Source: CAD feature listing. Evaluate the final solid. Frame: model axes, mm. A direction names the side the tool comes from. Give positions to 0.01 mm unless a question says otherwise; leave off trailing zeros. Order: outer loops, then holes, each group sorted by start corner. A loop starts at its lowest first (then second) coordinate and runs counter-clockwise, first axis right, second up.
from build123d import *

# Parameters (mm, degrees)
F2_R     = 20
F3_DEPTH = 20
F5_DEPTH = 15


with BuildPart() as f1:
    # F0 (on Front) → F1 (revolve)
    with BuildSketch(Plane.XZ):
        Polygon((29.861114, 20), (9.861114, 20), (9.861114, 65.476191), (29.861114, 65.476191), (29.861114, 90.476191), (0, 90.476191), (0, 0), (29.861114, 0), align=None)
    revolve(axis=Axis((0, 0, 45.238095), (0, 0, -1)))

    # F2 (on face) → F3 (cut)
    with BuildSketch(Plane.XY.offset(90.476191)):
        Circle(F2_R)
    extrude(amount=-F3_DEPTH, mode=Mode.SUBTRACT)

    # F4 (on face) → F5 (cut)
    with BuildSketch(Plane.XY.offset(90.476191)):
        with BuildLine():
            ThreePointArc((-3.013717, 17.091636), (0, 17.355302), (3.013717, 17.091636))
            Line((3.013717, 17.091636), (6.241417, 35.396835))
            ThreePointArc((6.241417, 35.396835), (0, 35.942888), (-6.241417, 35.396835))
            Line((-6.241417, 35.396835), (-3.013717, 17.091636))
        make_face()
        with BuildLine():
            Line((-33.775267, 12.293192), (-16.308649, 5.935863))
            ThreePointArc((-16.308649, 5.935863), (-15.030132, 8.677651), (-13.294933, 11.155773))
            Line((-13.294933, 11.155773), (-27.53385, 23.103643))
            ThreePointArc((-27.53385, 23.103643), (-31.127454, 17.971444), (-33.775267, 12.293192))
        make_face()
        with BuildLine():
            Line((-27.53385, -23.103643), (-13.294933, -11.155773))
            ThreePointArc((-13.294933, -11.155773), (-15.030132, -8.677651), (-16.308649, -5.935863))
            Line((-16.308649, -5.935863), (-33.775267, -12.293192))
            ThreePointArc((-33.775267, -12.293192), (-31.127454, -17.971444), (-27.53385, -23.103643))
        make_face()
        with BuildLine():
            Line((6.241417, -35.396835), (3.013717, -17.091636))
            ThreePointArc((3.013717, -17.091636), (0, -17.355302), (-3.013717, -17.091636))
            Line((-3.013717, -17.091636), (-6.241417, -35.396835))
            ThreePointArc((-6.241417, -35.396835), (0, -35.942888), (6.241417, -35.396835))
        make_face()
        with BuildLine():
            Line((33.775267, -12.293192), (16.308649, -5.935863))
            ThreePointArc((16.308649, -5.935863), (15.030132, -8.677651), (13.294933, -11.155773))
            Line((13.294933, -11.155773), (27.53385, -23.103643))
            ThreePointArc((27.53385, -23.103643), (31.127454, -17.971444), (33.775267, -12.293192))
        make_face()
        with BuildLine():
            Line((27.53385, 23.103643), (13.294933, 11.155773))
            ThreePointArc((13.294933, 11.155773), (15.030132, 8.677651), (16.308649, 5.935863))
            Line((16.308649, 5.935863), (33.775267, 12.293192))
            ThreePointArc((33.775267, 12.293192), (31.127454, 17.971444), (27.53385, 23.103643))
        make_face()
    extrude(amount=-F5_DEPTH, mode=Mode.SUBTRACT)


solid = f1.part
(1) Draft query along Z for faces 4 (the flat face through (-24, 0, 90.476)), 5 (the flat face through (7.1, -7.1, 65.476)), 6 (the flat face through (4.317, 24.484, 83.081)). Return one class per face: +Z half, -Z half, draft (parallel to the pull), parting line (faces both ways), or undercut.
(2) Section A-A, the plane x = 12.5. Return loops of the section in (y, z), plus the area to 3 significant figures.
(3) Pin query (flat end, axial travel): pin 1 Ø10 at (y, z) = (10, 46.5) entering from -X; pin 2 Ø3.5 at (x, y) = (23.5, -12) entering from +Z; pin 3 Ø6 at (x, z) = (-11, 52) entering from -Y. Return the tip coordinate at first contact, or that it passes through.
(4) Section C-C, the plane y = 0. Return loops of the section in (x, z).
(5) Section B-B, the plane y = 14. Return loops of the section in (x, z), plus the area to 3 significant figures.
(6) Access query for faces 1 (the flat face through (-22, -13, 75.476)), 2 (the flat face through (19.15, 16.07, 83.08)), 3 (the cylindrical face through (-1.284, -9.777, 43.056)). Directions: +Z, -Z, +X, -X, +Y, -Y. A direction counts if a zero-diameter tool reaches every point of the face in a straight line with its end or side. Return the directions, or none.
(7) Section D-D, the plane x = 0. Return loops of the section in (y, z), plus the area to 3 significant figures.
(8) Line query: line 1 along Z through (x, y) = (-23, -10); line 2 along Z through (x, y) = (-12, -27); line 3 along X through (y, z) = (0, 82). Output: solid intervals per line, ascending.
Checks:
1. face 4: +Z half
1. face 5: undercut
1. face 6: draft
2. outline: (-27.12, 0) - (27.12, 0) - (27.12, 20) - (-27.12, 20) - close; (-27.12, 65.48) - (27.12, 65.48) - (27.12, 90.48) - (15.61, 90.48) - (15.61, 70.48) - (-15.61, 70.48) - (-15.61, 90.48) - (-27.12, 90.48) - close
2. area: 1,820 mm2
3. pin 1: stops at x = -8.5
3. pin 2: stops at z = 75.48
3. pin 3: stops at y = -5.77
4. outline: (-29.86, 0) - (29.86, 0) - (29.86, 20) - (9.86, 20) - (9.86, 65.48) - (29.86, 65.48) - (29.86, 90.48) - (20, 90.48) - (20, 70.48) - (-20, 70.48) - (-20, 90.48) - (-29.86, 90.48) - (-29.86, 65.48) - (-9.86, 65.48) - (-9.86, 20) - (-29.86, 20) - close
5. outline: (-26.38, 0) - (26.38, 0) - (26.38, 20) - (-26.38, 20) - close; (-26.38, 65.48) - (26.38, 65.48) - (26.38, 75.48) - (16.68, 75.48) - (16.68, 90.48) - (14.28, 90.48) - (14.28, 70.48) - (-14.28, 70.48) - (-14.28, 90.48) - (-16.68, 90.48) - (-16.68, 75.48) - (-26.38, 75.48) - close
5. area: 1,510 mm2
6. face 1: +Z
6. face 2: +Z, +X
6. face 3: none
7. outline: (-29.86, 0) - (29.86, 0) - (29.86, 20) - (9.86, 20) - (9.86, 65.48) - (29.86, 65.48) - (29.86, 75.48) - (20, 75.48) - (20, 70.48) - (-20, 70.48) - (-20, 75.48) - (-29.86, 75.48) - (-29.86, 65.48) - (-9.86, 65.48) - (-9.86, 20) - (-29.86, 20) - close
7. area: 2,490 mm2
8. line 1: z = 0 to 20, 65.48 to 75.48
8. line 2: z = 0 to 20, 65.48 to 90.48
8. line 3: x = -29.86 to -20, 20 to 29.86
